Check sheet for the drawn part. Datum: minimum x, y, z corner. Units: mm. Coordinates: 2 decimals unless noted, no trailing zeros. Write each loop counter-clockwise with the first axis right and the second up, starting at its lowest first coordinate (ties: lowest second). Pieces come first, ordered by that corner, then holes. Notation, with made-up numbers: (53.25, 22) - (83.25, 22) arc R7 cw to (83.25, 27) - close; hole circle Ø1 at (19.25, 88). An arc over 180 degrees is marked (long way). Use CSV: the item, a comma, the result in double quotes. Start each with the question number.
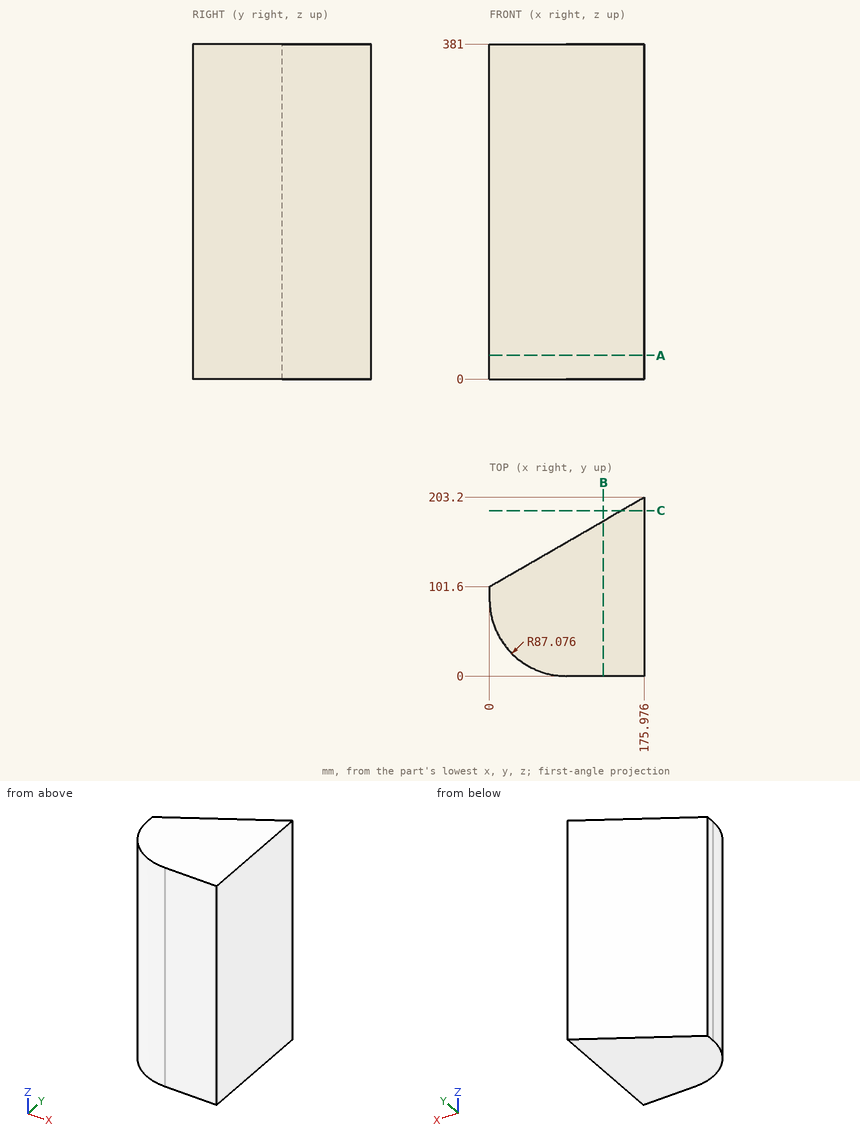
Q1. Scan lines: line 1 along X through (y, z) = (167.5, 257.5) (1 decimal); line 2 along Y through (x, z) = (22, 349); line 3 along Y through (x, z) = (154, 97.5). Record each from-to range of solid material in increasing order. Write a range as from..to.
Q2. Cross-section at B-B (x = 129.5). Record the cut outline in (y, z).
Q3. Cross-section at C-C (y = 188). Record the cut outline in (x, z), plus the area to 3 significant figures.
Q4. Gauge pin test, flat ends, axial feed: pin 1 (2 mm diameter, centred on y = 80.5, z = 46, fed in from -X); pin 2 (8 mm diameter, centred on x = 38, z = 250, fed in from -Y) (1 decimal); pin 3 (4 mm diameter, centred on y = 46, z = 75, fed in from -X). Record the tip position at first contact, or that the pin passes through.
Q5. Cross-section at A-A (z = 27). Record the cut outline in (x, y).
Reply:
1,line 1,"114.1..176"
1,line 2,"29.22..114.3"
1,line 3,"0..190.51"
2,outline,"(0, 0) - (176.37, 0) - (176.37, 381) - (0, 381) - close"
3,outline,"(149.65, 0) - (175.98, 0) - (175.98, 381) - (149.65, 381) - close"
3,area,"10,000 mm^2"
4,pin 1,"x = 0.18"
4,pin 2,"y = 12.6"
4,pin 3,"x = 9.26"
5,outline,"(0, 87.08) arc R87.08 ccw to (87.08, 0) - (175.98, 0) - (175.98, 203.2) - (0, 101.6) - close"
